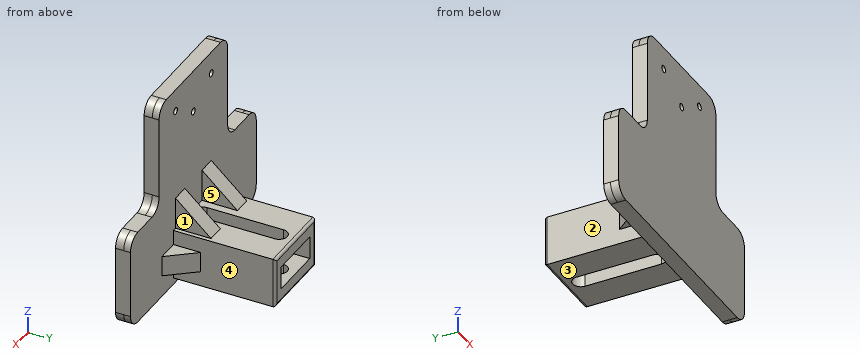
from build123d import *

# Parameters (mm, degrees)
EXTRUDE_1_DEPTH     = 6
SKETCH_2_W          = 40
SKETCH_2_H          = 17
EXTRUDE_2_DEPTH     = 80
EXTRUDE_3_DEPTH     = 7.5
EXTRUDE_4_DEPTH     = 25
CUT_EXTRUDE_1_DEPTH = 124.93663618022231
CUT_EXTRUDE_2_DEPTH = 80
FILLET_1_R          = 2
SKETCH_11_R         = 2.549999999999998
SKETCH_11_W         = 176.00000000000006
SKETCH_11_H         = 70
EXTRUDE_5_DEPTH     = 6
FILLET_2_R          = 10
EXTRUDE_6_OUTLINE_R = 2.55
EXTRUDE_6_DEPTH     = 5


# Read off the part's stored shape, not the designer's step: 凸台-拉伸6
with BuildPart() as part:
    # 草图1 → 凸台-拉伸1 (new body)
    with BuildSketch(Plane(origin=(0, 0, 0), x_dir=(1, 0, 0), z_dir=(0, 1, 0))):
        Polygon((-61.14973252328083, 43.789730909681225), (-61.149732523280825, -26.210269090318775), (34.85026747671919, -26.210269090318782), (34.85026747671917, 43.789730909681225), align=None)
    extrude(amount=EXTRUDE_1_DEPTH)

    # 草图2 → 凸台-拉伸2 (add)
    with BuildSketch(Plane(origin=(0, 6, 0), x_dir=(1, 0, 0), z_dir=(0, 1, 0))):
        Polygon((-41.14973252328083, 38.78973090968122), (14.850267476719164, 38.78973090968122), (14.850267476719166, 1.7897309096812228), (-41.149732523280825, 1.7897309096812228), align=None)
        with Locations((-13.14973252328083, 20.289730909681225)):
            Rectangle(SKETCH_2_W, SKETCH_2_H, mode=Mode.SUBTRACT)
    extrude(amount=EXTRUDE_2_DEPTH)

    # 草图5 → 凸台-拉伸3 (add, symmetric)
    with BuildSketch(Plane.XY.offset(-20.289730909681218)):
        Polygon((-61.14973252328082, 6), (-41.149732523280825, 31), (-41.14973252328082, 6), align=None)
        Polygon((14.850267476719168, 30.999999999999996), (34.850267476719196, 6), (14.85026747671917, 6), align=None)
    extrude(amount=EXTRUDE_3_DEPTH, both=True)

    # 草图8 → 凸台-拉伸4 (add, symmetric)
    with BuildSketch(Plane(origin=(-13.149732523280829, 0, -1.23e-15), x_dir=(9e-17, 0, -1), z_dir=(1, 0, 9e-17))):
        Polygon((-26.21026909031878, 6), (1.7897309096812217, 37.0606214388455), (1.7897309096812242, 6), align=None)
    extrude(amount=EXTRUDE_4_DEPTH, both=True)

    # 草图9 → 切除-拉伸1 (cut, through all)
    with BuildSketch(Plane(origin=(0, 0, -38.78973090968122), x_dir=(-1, 0, 0), z_dir=(0, 0, -1))):
        with BuildLine():
            Line((19.149732523280832, 74.00000000000001), (19.149732523280832, 18.000000000000004))
            ThreePointArc((19.149732523280832, 18.000000000000004), (13.149732523280827, 12.000000000000002), (7.149732523280827, 18.000000000000004))
            Line((7.149732523280827, 18.000000000000004), (7.149732523280827, 74.00000000000001))
            ThreePointArc((7.149732523280827, 74.00000000000001), (13.149732523280829, 80.00000000000001), (19.149732523280832, 74.00000000000001))
        make_face()
    extrude(amount=-CUT_EXTRUDE_1_DEPTH, mode=Mode.SUBTRACT)

    # 草图10 → 切除-拉伸2 (cut)
    with BuildSketch(Plane(origin=(0, 86, 0), x_dir=(1, 0, 0), z_dir=(0, 1, 0))):
        Polygon((-25.14973252328083, 1.7897309096812328), (-1.1497325232808289, 1.7897309096812328), (-1.1497325232808246, -29.118616684918184), (-25.149732523280825, -29.118616684918184), align=None)
    extrude(amount=-CUT_EXTRUDE_2_DEPTH, mode=Mode.SUBTRACT)

    # 圆角1
    fillet_1_edges = [part.edges().sort_by_distance(p)[0] for p in [
        (14.850267476719164, 86, -20.28973090968122),
        (-13.149732523280832, 86, -38.78973090968122),
        (-41.14973252328083, 86, -20.289730909681218),
        (-13.14973252328083, 86, -1.7897309096812228),
    ]]
    fillet(fillet_1_edges, radius=FILLET_1_R)

    # 草图11 → 凸台-拉伸5 (add)
    # profile 1 of 3: a face of its own
    with BuildSketch(Plane.XZ):
        Polygon((-61.14973252328083, -43.789730909681225), (34.85026747671919, -43.789730909681225), (34.850267476719196, 106.21026909031877), (-61.14973252328083, 106.21026909031877), align=None)
        with Locations(Location((-38.14973252328083, 89.71026909031877, 0), (0, 0, 270))):
            Circle(SKETCH_11_R, mode=Mode.SUBTRACT)
        with Locations(Location((11.850267476719166, 89.71026909031877, 0), (0, 0, 270))):
            Circle(SKETCH_11_R, mode=Mode.SUBTRACT)
        with Locations(Location((-13.149732523280832, 74.71026909031877, 0), (0, 0, 270))):
            Circle(SKETCH_11_R, mode=Mode.SUBTRACT)
    # profile 2 of 3: a face of its own
    with BuildSketch(Plane.XZ):
        with Locations((-13.149732523280825, -8.789730909681222)):
            Rectangle(SKETCH_11_W, SKETCH_11_H)
    # profile 3 of 3: a face of its own
    with BuildSketch(Plane.XZ):
        Polygon((12.850267476719164, -36.78973090968122), (12.850267476719166, -3.789730909681223), (-39.14973252328082, -3.789730909681223), (-39.149732523280825, -36.78973090968122), align=None)
    extrude(amount=-EXTRUDE_5_DEPTH)

    # 圆角2
    fillet_2_edges = [part.edges().sort_by_distance(p)[0] for p in [
        (-61.149732523280825, 3, 26.21026909031878),
        (-61.14973252328083, 3, 106.21026909031877),
        (34.850267476719196, 3, 106.21026909031877),
        (34.85026747671919, 3, 26.21026909031878),
        (74.8502674767192, 3, 26.210269090318782),
        (74.8502674767192, 3, -43.789730909681225),
        (-101.14973252328083, 3, -43.789730909681225),
        (-101.14973252328083, 3, 26.210269090318782),
    ]]
    fillet(fillet_2_edges, radius=FILLET_2_R)

    # 凸台-拉伸6 outline → 凸台-拉伸6 (add)
    with BuildSketch(Plane(origin=(0, 6, 0), x_dir=(1, 0, 0), z_dir=(0, 1, 0))):
        with BuildLine():
            ThreePointArc((-61.149732523, -96.21026909), (-58.220800335, -103.281336902), (-51.149732523, -106.21026909))
            Line((-51.149732523, -106.21026909), (24.850267477, -106.21026909))
            ThreePointArc((24.850267477, -106.21026909), (31.921335289, -103.281336902), (34.850267477, -96.21026909))
            Line((34.850267477, -96.21026909), (34.850267477, -36.21026909))
            ThreePointArc((34.850267477, -36.21026909), (37.779199665, -29.139201278), (44.850267477, -26.21026909))
            Line((44.850267477, -26.21026909), (64.850267477, -26.21026909))
            ThreePointArc((64.850267477, -26.21026909), (71.921335289, -23.281336902), (74.850267477, -16.21026909))
            Line((74.850267477, -16.21026909), (74.850267477, 33.78973091))
            ThreePointArc((74.850267477, 33.78973091), (71.921335289, 40.860798722), (64.850267477, 43.78973091))
            Line((64.850267477, 43.78973091), (-91.149732523, 43.78973091))
            ThreePointArc((-91.149732523, 43.78973091), (-98.220800335, 40.860798722), (-101.149732523, 33.78973091))
            Line((-101.149732523, 33.78973091), (-101.149732523, -16.21026909))
            ThreePointArc((-101.149732523, -16.21026909), (-98.220800335, -23.281336902), (-91.149732523, -26.21026909))
            Line((-91.149732523, -26.21026909), (-71.149732523, -26.21026909))
            ThreePointArc((-71.149732523, -26.21026909), (-64.078664711, -29.139201278), (-61.149732523, -36.21026909))
            Line((-61.149732523, -36.21026909), (-61.149732523, -96.21026909))
        make_face()
        with Locations((-38.149732523, -89.71026909)):
            Circle(EXTRUDE_6_OUTLINE_R, mode=Mode.SUBTRACT)
        with Locations((11.850267477, -89.71026909)):
            Circle(EXTRUDE_6_OUTLINE_R, mode=Mode.SUBTRACT)
        with Locations((-13.149732523, -74.71026909)):
            Circle(EXTRUDE_6_OUTLINE_R, mode=Mode.SUBTRACT)
    extrude(amount=EXTRUDE_6_DEPTH)


solid = part.part
Work out the finished part from the listing and answer in its coordinate system (mm). Face numbers are marked on the shaded views. A direction names the side the tool comes from. Round coordinates to 2 decimals unless told otherwise and drop trailing zeros. Loops run counter-clockwise (first coordinate to the right, second up) from the corner with the lowest first, then second, coordinate; pieces in that order, holes last. Notation, with made-up numbers: M 76.5,-32 L 82.5,-32 A23 ccw 82.5,-8 Z; hole C 40.5,89 d9. An arc over 180 degrees is marked long. One line per question, with ' | ' between items. Start each with the question number.
(1) A cutting plane is placed at D-D on y = 78. Write down the section's boundary in (x, z).
(2) Find the intervals of material crossed by line 1 (Z direction, x = -5.5, y = 52); line 2 (X direction, y = 50, z = -13.5); line 3 (X direction, y = 7, z = 48.5), in increasing order.
(3) A cutting plane is placed at C-C on x = 27.5. Write down the section's boundary in (y, z).
(4) A cutting plane is placed at B-B on z = 19.5. Write down the section's boundary in (x, y), plus the area to 3 significant figures.
(5) A cutting plane is placed at A-A on y = 59. Write down the section's boundary in (x, z), plus the area to 3 significant figures.
(6) Flat-ended cylindrical pins translate along their axes: pin 1 Ø1.5 at (x, z) = (-71, -22.5) entering from +Y; pin 2 Ø4 at (y, z) = (75, -11.5) entering from +X; pin 3 Ø13 at (x, y) = (25.5, 24.5) entering from -Z. Find the tip coordinate at first contact, or state that the pin passes through.
(7) A tool of negligible diameter and unlimited length cuts with its end or side. For the marked faces 1, 2, 3, 4 and 5, from which of +Z, -Z, +X, -X, +Y, -Y can it reach the whole face along a straight path? Write none if from no direction.
Geometry check:
1) outline: M -41.15,-38.79 L -17.62,-38.79 L -17.62,-28.79 L -33.15,-28.79 L -33.15,-11.79 L -17.62,-11.79 L -17.62,-1.79 L -41.15,-1.79 Z; M -8.68,-38.79 L 14.85,-38.79 L 14.85,-1.79 L -8.68,-1.79 L -8.68,-11.79 L 6.85,-11.79 L 6.85,-28.79 L -8.68,-28.79 Z
2) line 1: z = -38.79 to -28.79, -11.79 to -1.79 | line 2: x = -41.15 to -33.15, 6.85 to 14.85 | line 3: x = -61.15 to 34.85
3) outline: M 0,-43.79 L 11,-43.79 L 11,-27.79 L 15.19,-27.79 L 15.19,-12.79 L 11,-12.79 L 11,105.85 L 0,105.85 Z
4) outline: M -100.59,0 L 74.29,0 L 74.29,11 L 11.85,11 L 11.85,13.44 L -1.15,13.44 L -1.15,11 L -25.15,11 L -25.15,13.44 L -38.15,13.44 L -38.15,11 L -100.59,11 Z | area: 1,990 mm²
5) outline: M -41.15,-38.79 L -19.15,-38.79 L -19.15,-28.79 L -33.15,-28.79 L -33.15,-11.79 L -19.15,-11.79 L -19.15,-1.79 L -41.15,-1.79 Z; M -7.15,-38.79 L 14.85,-38.79 L 14.85,-1.79 L -7.15,-1.79 L -7.15,-11.79 L 6.85,-11.79 L 6.85,-28.79 L -7.15,-28.79 Z | area: 1,150 mm²
6) pin 1: stops at y = 11 | pin 2: stops at x = 14.85 | pin 3: stops at z = -27.79
7) face 1: +Z, +X, +Y | face 2: -X, +Y | face 3: -Z, +X, -X, +Y | face 4: +X, +Y | face 5: +Z, +Y
